from build123d import *

# Parameters (mm, degrees)
BOSS_EXTRUDE1_DEPTH = 2
FILLET1_R           = 80
SKETCH4_R           = 1.5
CUT_EXTRUDE1_DEPTH  = 10
CUT_EXTRUDE2_DEPTH  = 10
FILLET2_R           = 2
CUT_EXTRUDE3_DEPTH  = 10
CUT_EXTRUDE4_DEPTH  = 10
SKETCH8_R           = 1
CUT_EXTRUDE5_DEPTH  = 10
SKETCH9_R           = 1.5
CUT_EXTRUDE6_DEPTH  = 10


with BuildPart() as part:
    # Sketch1 → Boss-Extrude1 (new body)
    with BuildSketch(Plane(origin=(0, 0, 0), x_dir=(1, 0, 0), z_dir=(0, 1, 0))):
        Polygon((-88, 41.502433661), (-88, -41.502433661), (-120.139380484, -79.804655817), (-93.327824975, -102.302222156), (-61.188444491, -64), (61.188444491, -64), (93.327824975, -102.302222156), (120.139380484, -79.804655817), (88, -41.502433661), (88, 41.502433661), (120.139380484, 79.804655817), (93.327824975, 102.302222156), (61.188444491, 64), (-61.188444491, 64), (-93.327824975, 102.302222156), (-120.139380484, 79.804655817), align=None)
    extrude(amount=BOSS_EXTRUDE1_DEPTH)

    # Fillet1
    fillet1_edges = [part.edges().sort_by_distance(p)[0] for p in [
        (61.188444491, 1, -64),
        (88, 1, -41.502433661),
        (88, 1, 41.502433661),
        (61.188444491, 1, 64),
        (-61.188444491, 1, 64),
        (-88, 1, 41.502433661),
        (-88, 1, -41.502433661),
        (-61.188444491, 1, -64),
    ]]
    fillet(fillet1_edges, radius=FILLET1_R)

    # Sketch4 → Cut-Extrude1 (cut)
    with BuildSketch(Plane(origin=(0, 2, 0), x_dir=(1, 0, 0), z_dir=(0, 1, 0))):
        with Locations(Location((-101.591301852, -84.925083441, 0), (0, 0, 270))):
            Circle(SKETCH4_R)
        with Locations(Location((-82.950461171, -62.709794591, 0), (0, 0, 270))):
            Circle(SKETCH4_R)
        with Locations(Location((101.591301852, -84.925083441, 0), (0, 0, 270))):
            Circle(SKETCH4_R)
        with Locations(Location((82.950461171, -62.709794591, 0), (0, 0, 270))):
            Circle(SKETCH4_R)
        with Locations(Location((101.591301852, 84.925083441, 0), (0, 0, 270))):
            Circle(SKETCH4_R)
        with Locations(Location((82.950461171, 62.709794591, 0), (0, 0, 270))):
            Circle(SKETCH4_R)
        with Locations(Location((-101.591301852, 84.925083441, 0), (0, 0, 270))):
            Circle(SKETCH4_R)
        with Locations(Location((-82.950461171, 62.709794591, 0), (0, 0, 270))):
            Circle(SKETCH4_R)
    extrude(amount=-CUT_EXTRUDE1_DEPTH, mode=Mode.SUBTRACT)

    # Sketch5 → Cut-Extrude2 (cut)
    with BuildSketch(Plane(origin=(0, 2, 0), x_dir=(1, 0, 0), z_dir=(0, 1, 0))):
        Polygon((-30, 30), (30, 30), (58.562960135, 50), (-58.562960135, 50), align=None)
        Polygon((-58.562960135, -50), (-30, -30), (30, -30), (58.562960135, -50), align=None)
        Polygon((-50, 20), (-50, -20), (-75, -37.505188455), (-75, 37.505188455), align=None)
        Polygon((75, 37.505188455), (50, 20), (50, -20), (75, -37.505188455), align=None)
    extrude(amount=-CUT_EXTRUDE2_DEPTH, mode=Mode.SUBTRACT)

    # Fillet2
    fillet2_edges = [part.edges().sort_by_distance(p)[0] for p in [
        (50, 1, -20),
        (75, 1, -37.505188455),
        (75, 1, 37.505188455),
        (50, 1, 20),
        (-30, 1, 30),
        (30, 1, 30),
        (58.562960135, 1, 50),
        (-58.562960135, 1, 50),
        (-58.562960135, 1, -50),
        (58.562960135, 1, -50),
        (30, 1, -30),
        (-30, 1, -30),
        (-75, 1, -37.505188455),
        (-50, 1, -20),
        (-50, 1, 20),
        (-75, 1, 37.505188455),
    ]]
    fillet(fillet2_edges, radius=FILLET2_R)

    # Sketch5<3> → Cut-Extrude3 (cut)
    with BuildSketch(Plane(origin=(0, 2, 0), x_dir=(1, 0, 0), z_dir=(0, 1, 0))):
        with BuildLine():
            Line((-15, -13.770980054), (-15, -15))
            Line((-15, -15), (-13.770980054, -15))
            ThreePointArc((-13.770980054, -15), (-14.189339828, -14.189339828), (-15, -13.770980054))
        make_face()
        with BuildLine():
            Line((-13.770980054, -15), (-15, -15))
            Line((-15, -15), (-15, -13.770980054))
            ThreePointArc((-15, -13.770980054), (-16.395643924, -16.218245837), (-13.75, -15.25))
            ThreePointArc((-13.75, -15.25), (-13.755254216, -15.12456061), (-13.770980054, -15))
        make_face()
        with BuildLine():
            ThreePointArc((15, -13.770980054), (14.189339828, -14.189339828), (13.770980054, -15))
            Line((13.770980054, -15), (15, -15))
            Line((15, -15), (15, -13.770980054))
        make_face()
        with BuildLine():
            Line((15, -15), (13.770980054, -15))
            ThreePointArc((13.770980054, -15), (15.12456061, -16.744745784), (16.75, -15.25))
            ThreePointArc((16.75, -15.25), (16.218245837, -14.104356076), (15, -13.770980054))
            Line((15, -13.770980054), (15, -15))
        make_face()
        with BuildLine():
            ThreePointArc((13.770980054, 15), (14.189339828, 14.189339828), (15, 13.770980054))
            Line((15, 13.770980054), (15, 15))
            Line((15, 15), (13.770980054, 15))
        make_face()
        with BuildLine():
            Line((15, 15), (15, 13.770980054))
            ThreePointArc((15, 13.770980054), (16.218245837, 14.104356076), (16.75, 15.25))
            ThreePointArc((16.75, 15.25), (15.12456061, 16.744745784), (13.770980054, 15))
            Line((13.770980054, 15), (15, 15))
        make_face()
        with BuildLine():
            ThreePointArc((-13.75, 15.25), (-16.395643924, 16.218245837), (-15, 13.770980054))
            Line((-15, 13.770980054), (-15, 15))
            Line((-15, 15), (-13.770980054, 15))
            ThreePointArc((-13.770980054, 15), (-13.755254216, 15.12456061), (-13.75, 15.25))
        make_face()
        with BuildLine():
            Line((-15, 15), (-15, 13.770980054))
            ThreePointArc((-15, 13.770980054), (-14.189339828, 14.189339828), (-13.770980054, 15))
            Line((-13.770980054, 15), (-15, 15))
        make_face()
    extrude(amount=-CUT_EXTRUDE3_DEPTH, mode=Mode.SUBTRACT)

    # Sketch6 → Cut-Extrude4 (cut)
    with BuildSketch(Plane(origin=(0, 2, 0), x_dir=(1, 0, 0), z_dir=(0, 1, 0))):
        with BuildLine():
            Line((-10.5, -12.5), (10.5, -12.5))
            ThreePointArc((10.5, -12.5), (11.914213562, -11.914213562), (12.5, -10.5))
            Line((12.5, -10.5), (12.5, 10.5))
            ThreePointArc((12.5, 10.5), (11.914213562, 11.914213562), (10.5, 12.5))
            Line((10.5, 12.5), (-10.5, 12.5))
            ThreePointArc((-10.5, 12.5), (-11.914213562, 11.914213562), (-12.5, 10.5))
            Line((-12.5, 10.5), (-12.5, -10.5))
            ThreePointArc((-12.5, -10.5), (-11.914213562, -11.914213562), (-10.5, -12.5))
        make_face()
    extrude(amount=-CUT_EXTRUDE4_DEPTH, mode=Mode.SUBTRACT)

    # Sketch8 → Cut-Extrude5 (cut)
    with BuildSketch(Plane.XZ):
        with Locations(Location((64, 35.5, 0), (0, 0, 270))):
            Circle(SKETCH8_R)
        with Locations(Location((64, 62.5, 0), (0, 0, 270))):
            Circle(SKETCH8_R)
        with Locations(Location((-64, 62.5, 0), (0, 0, 270))):
            Circle(SKETCH8_R)
        with Locations(Location((-64, 35.5, 0), (0, 0, 270))):
            Circle(SKETCH8_R)
        with Locations(Location((-64, -62.5, 0), (0, 0, 270))):
            Circle(SKETCH8_R)
        with Locations(Location((-64, -35.5, 0), (0, 0, 270))):
            Circle(SKETCH8_R)
        with Locations(Location((64, -35.5, 0), (0, 0, 270))):
            Circle(SKETCH8_R)
        with Locations(Location((64, -62.5, 0), (0, 0, 270))):
            Circle(SKETCH8_R)
    extrude(amount=-CUT_EXTRUDE5_DEPTH, mode=Mode.SUBTRACT)

    # Sketch9 → Cut-Extrude6 (cut)
    with BuildSketch(Plane(origin=(0, 2, 0), x_dir=(1, 0, 0), z_dir=(0, 1, 0))):
        with Locations(Location((48.5, 31.293024341, 0), (0, 0, 270))):
            Circle(SKETCH9_R)
        with Locations(Location((48.5, -31.293024341, 0), (0, 0, 270))):
            Circle(SKETCH9_R)
        with Locations(Location((-48.5, -36.293024341, 0), (0, 0, 270))):
            Circle(SKETCH9_R)
        with Locations(Location((-48.5, 36.293024341, 0), (0, 0, 270))):
            Circle(SKETCH9_R)
    extrude(amount=-CUT_EXTRUDE6_DEPTH, mode=Mode.SUBTRACT)


solid = part.part
Can you work these out from the model? Positions are in its coordinate system, mm. A direction names the side the tool comes from. Coordinates: 2 decimals unless noted, no trailing zeros. Loops run counter-clockwise (first coordinate to the right, second up) from the corner with the lowest first, then second, coordinate; pieces in that order, holes last. Notation, with made-up numbers: M -11,86.25 L 47,86.25 A19 ccw 47,116.25 Z; hole C 26.25,58.25 d4. An arc over 180 degrees is marked long. Answer as CSV lines item,"result". Start each with the question number.
1. Suppose I cut it at D-D, the plane y = 1.35. Count the separate pieces of the cut face and the enclosed holes in it, plus the area to 3 significant figures.
2. For faces 1 (the face through (-92.7, 1, -39.4)), 2 (the face through (61.21, 1.01, 27.85)), 3 (the face through (-58.136, 1.014, 71.703)), which set-ups out of +Z, -Z, +X, -X, +Y, -Y let a thin tool reach every point of the face, with its end or its side?
3. If I drill on probe 1 along Z at (x, y) = (-26.5, 1.7); probe 2 along X at (y, z) = (1.4, 15.25); probe 3 along X at (y, z) = (1.75, -7), over which ranges is the centre line in solid material (lowest first)? Write a range as [from, to].
4. For pin 1 Ø0.6 at (y, z) = (0.5, -1) entering from +X; pin 2 Ø1 at (y, z) = (1, 35.5) entering from +X, each with a flat end and sliding along its axis, tell me the tip position at first contact or that it passes through.
5. Suppose I cut it at B-B, the plane x = -39. List the corners of the cut face in (y, z) for me, plus the area to 3 significant figures.
6. Suppose I cut it at C-C, the plane z = 27. List the corners of the cut face in (x, y) for me, plus the area to 3 significant figures.
7. Suppose I cut it at A-A, the plane z = -43. List the corners of the cut face in (x, y) for me.
8. Thinking about a two-plate mould opening in X: for faces 4 (the face through (-57.25, 1.01, -71.29)), 5 (the face through (-106.921, 0.986, 90.896)), 6 (the face through (89.19, 0.99, 97.37)), 7 (the face through (-2, 0, 21)), which applies, +X half, -X half, draft (parallel to the pull), parting line (faces both ways), or undercut?
Output:
1,separate pieces,"1"
1,enclosed holes,"29"
1,area,"22,300 mm^2"
2,face 1,"-X, +Y, -Y"
2,face 2,"+Y, -Y"
2,face 3,"+Z, +Y, -Y"
3,probe 1,"z = [-64.04, -50], [-30, 30], [50, 64.04]"
3,probe 2,"x = [-88.05, -75], [-50, -16.75], [-13.75, 13.75], [16.75, 50], [75, 88.05]"
3,probe 3,"x = [-88, -75], [-50, -12.5], [12.5, 50], [75, 88]"
4,pin 1,"stops at x = 88"
4,pin 2,"stops at x = 91.56"
5,outline,"M 0,-65.44 L 2,-65.44 L 2,-50 L 0,-50 Z; M 0,-36.3 L 2,-36.3 L 2,36.3 L 0,36.3 Z; M 0,50 L 2,50 L 2,65.44 L 0,65.44 Z"
5,area,"207 mm^2"
6,outline,"M -89.35,0 L -75,0 L -75,2 L -89.35,2 Z; M -60,0 L 60,0 L 60,2 L -60,2 Z; M 75,0 L 89.35,0 L 89.35,2 L 75,2 Z"
6,area,"297 mm^2"
7,outline,"M -94.09,0 L -48.57,0 L -48.57,2 L -94.09,2 Z; M 48.57,0 L 94.09,0 L 94.09,2 L 48.57,2 Z"
8,face 4,"undercut"
8,face 5,"-X half"
8,face 6,"undercut"
8,face 7,"draft"
